Can you work these out from the drawing? Everything is in mm from the part's minimum corner. A direction names the side the tool comes from. Coordinates: 2 decimals unless noted, no trailing zeros. Loops run counter-clockwise (first coordinate to the right, second up) from the corner with the lowest first, then second, coordinate; pieces in that order, holes last. Notation, with made-up numbers: (60.25, 32) -> (107.25, 32) arc R14 ccw to (107.25, 43) -> close; hole circle Ø7 at (31, 76.5). An arc over 180 degrees is marked (long way). One line per question, with ' | ' between items.
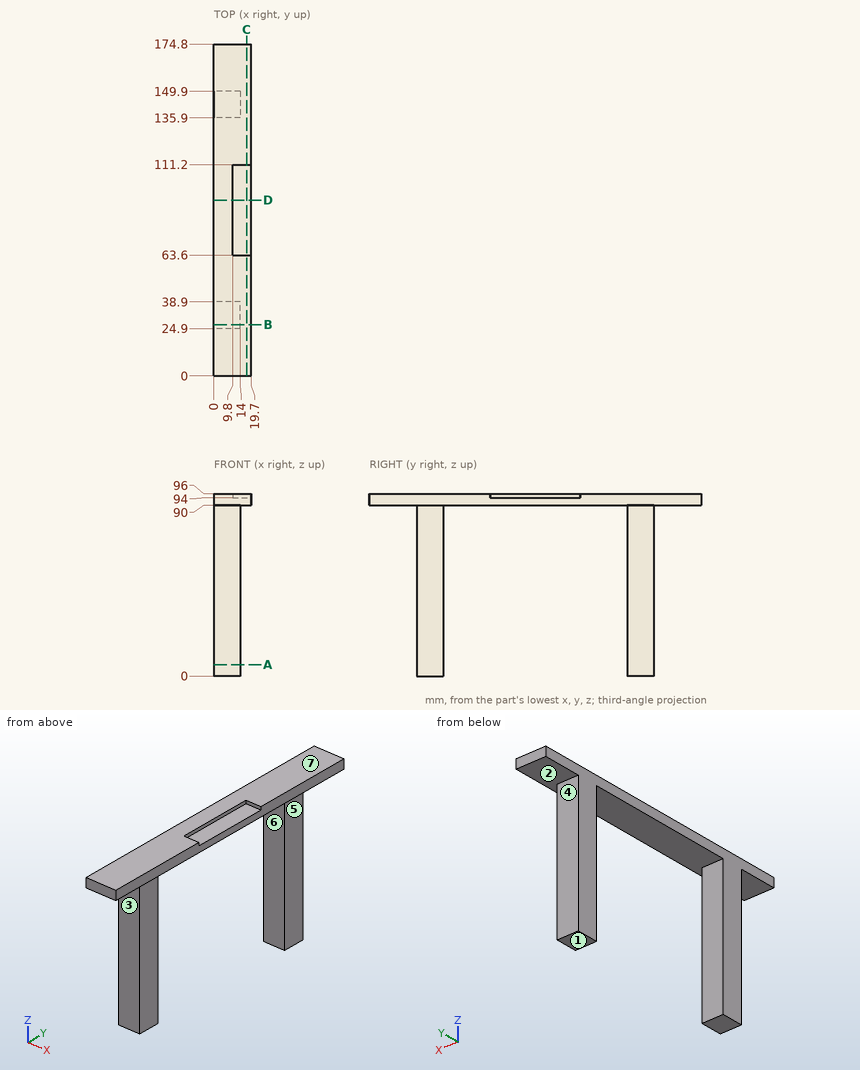
Q1. Imagine slicing it at C-C on x = 17.25. Write out the boundary of the cut face in (y, z), plus the area to 3 significant figures.
Values follow:
outline: (0, 90) -> (174.8, 90) -> (174.8, 96) -> (111.2, 96) -> (111.2, 94) -> (63.6, 94) -> (63.6, 96) -> (0, 96) -> close | area: 954 mm2
Q2. Imagine slicing it at D-D on y = 92.5. Write out the boundary of the cut face in (x, z), plus the area to 3 significant figures.
Values follow:
outline: (0, 90) -> (19.7, 90) -> (19.7, 94) -> (9.8, 94) -> (9.8, 96) -> (0, 96) -> close | area: 98.4 mm2
Q3. For pin 1 (15.5 mm diameter, centred on y = 140.5, z = 65, fed in from +X); pin 2 (11 mm diameter, centred on x = 7.5, z = 49.5, fed in from +Y); pin 3 (4 mm diameter, centred on x = 6, z = 39.5, fed in from -Y), each with a flat end and sliding along its axis, tell me the tip position at first contact or that it passes through.
Values follow:
pin 1: stops at x = 14 | pin 2: stops at y = 149.9 | pin 3: stops at y = 24.9
Q4. We'd pull the mould along Y, two halves only. Please class the marked faces 1, 2, 3 and 4: released by +Y, released by -Y, zero draft, split by the parting line, or undercut.
Values follow:
face 1: zero draft | face 2: undercut | face 3: released by -Y | face 4: released by +Y
Q5. Imagine slicing it at B-B on y = 27. Write out the boundary of the cut face in (x, z).
Values follow:
outline: (0, 0) -> (14, 0) -> (14, 90) -> (19.7, 90) -> (19.7, 96) -> (0, 96) -> close
Q6. Imagine slicing it at A-A on z = 6. Write out the boundary of the cut face in (x, y).
Values follow:
outline: (0, 24.9) -> (14, 24.9) -> (14, 38.9) -> (0, 38.9) -> close; (0, 135.9) -> (14, 135.9) -> (14, 149.9) -> (0, 149.9) -> close
Q7. For the marked faces 5, 6 and 7, which set-ups out of +Z, -Z, +X, -X, +Y, -Y let a thin tool reach every point of the face, with its end or its side?
Values follow:
face 5: -Z, +X, +Y, -Y | face 6: -Z, +X, -X | face 7: +Z, +X, -X, +Y, -Y
Q8. Please list where these lines run through material, in increasing order: L1, parallel to Y at x = 5.75, z = 21.5; L2, parallel to Z at x = 17, y = 103.5; L3, parallel to X at y = 136.5, z = 44. Write a range as [from, to].
Values follow:
L1: y = [24.9, 38.9], [135.9, 149.9] | L2: z = [90, 94] | L3: x = [0, 14]
